Geometry: final body of the model. Coordinates: model frame, mm. Face numbers are marked on the shaded views. A direction names the side the tool comes from. Give positions to 0.01 mm unless a question says otherwise; leave off trailing zeros. Order: outer loops, then holes, each group sorted by start corner. A loop starts at its lowest first (then second) coordinate and runs counter-clockwise, first axis right, second up. Notation, with made-up numbers: (4.5, 16.25) - (52.5, 16.25) arc R13 cw to (52.5, 24.25) - close; hole circle Ø5 at (-1, 53.25). An arc over 180 degrees is marked (long way). Write item = value, one per line. Start each with the question number.
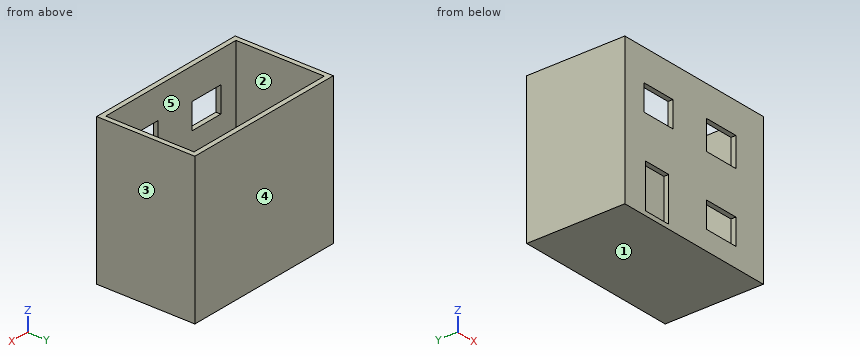
from build123d import *

# Parameters (mm, degrees)
F0_W     = 85.893087
F0_H     = 76.244824
F1_DEPTH = 50.8
F2_T     = -2.54
F3_W     = 17.883054
F3_H     = 13.338813
F3_W_2   = 18.097924
F3_H_2   = 15.061585
F3_H_3   = 13.338815
F3_W_3   = 14.340789
F3_H_4   = 22.664875
F4_DEPTH = 25.4


with BuildPart() as f1:
    # F0 (on Front) → F1 (new body)
    with BuildSketch(Plane.XZ):
        with Locations((2.00025, -38.122412)):
            Rectangle(F0_W, F0_H)
    extrude(amount=F1_DEPTH)

    # F2
    f2_openings = [f1.faces().sort_by_distance(p)[0] for p in [
        (2.00025, -25.4, 0),
    ]]
    offset(amount=F2_T, openings=f2_openings)

    # F3 (on face) → F4 (cut)
    with BuildSketch(Plane.XZ.offset(50.8)):
        with Locations((-20.056449, -22.847423)):
            Rectangle(F3_W, F3_H)
        with Locations((18.888849, -23.377542)):
            Rectangle(F3_W_2, F3_H_2)
        with Locations((18.888849, -59.610495)):
            Rectangle(F3_W_2, F3_H_3)
        with Locations((-20.887177, -62.660388)):
            Rectangle(F3_W_3, F3_H_4)
    extrude(amount=-F4_DEPTH, mode=Mode.SUBTRACT)


solid = f1.part
Q1. Contact query for a flat-ended pin moving along its axis: pin 1 (4.5 mm diameter, centred on x = -20.5, y = -34, fed in from +Z). Output: stop coordinate, or through.
Q2. Material intervals for line 1 along X through (y, z) = (-10, -23); line 2 along Y through (x, z) = (9, -44); line 3 along Z through (x, y) = (-17.5, -26.5), sorted ascending. Write a range as from..to.
Q3. Section A-A, the plane x = 13. Return the cut outline in (y, z).
Q4. Section B-B, the plane z = -62. Return the cut outline in (x, y), then the cut area to 3 significant figures.
Q5. Section C-C, the plane y = -23. Return the cut outline in (x, z).
Q6. Set-up query: the marked faces 1 and 2. Return all of +Z, -Z, +X, -X, +Y, -Y with unobstructed straight access to the full face (end or side cutting, diameter ignored); none if empty.
Q7. Pull-direction query (Y, two-part tool) for the marked faces 3, 4 and 5; classes: +Y half, -Y half, draft (parallel to the pull), parting line (faces both ways), or undercut.
Q8. Section D-D, the plane x = -5.5. Return the cut outline in (y, z).
The answers:
q1.pin_1 = -73.99
q2.line_1 = -40.95..-38.41, 42.41..44.95
q2.line_2 = -50.8..-48.26, -2.54..0
q2.line_3 = -76.24..-73.99
q3.outline = (-50.8, -76.24) - (0, -76.24) - (0, 0) - (-2.54, 0) - (-2.54, -73.7) - (-48.26, -73.7) - (-48.26, -66.28) - (-50.8, -66.28) - close; (-50.8, -52.94) - (-48.26, -52.94) - (-48.26, -30.91) - (-50.8, -30.91) - close; (-50.8, -15.85) - (-48.26, -15.85) - (-48.26, 0) - (-50.8, 0) - close
q4.outline = (-40.95, -50.8) - (-28.06, -50.8) - (-28.06, -48.26) - (-38.41, -48.26) - (-38.41, -2.54) - (42.41, -2.54) - (42.41, -48.26) - (27.94, -48.26) - (27.94, -50.8) - (44.95, -50.8) - (44.95, 0) - (-40.95, 0) - close; (-13.72, -50.8) - (9.84, -50.8) - (9.84, -48.26) - (-13.72, -48.26) - close
q4.area = 586 mm²
q5.outline = (-40.95, -76.24) - (44.95, -76.24) - (44.95, 0) - (42.41, 0) - (42.41, -73.7) - (-38.41, -73.7) - (-38.41, 0) - (-40.95, 0) - close
q6.face_1 = -Z, +X, -X, +Y, -Y
q6.face_2 = +Z
q7.face_3 = draft
q7.face_4 = +Y half
q7.face_5 = undercut
q8.outline = (-50.8, -76.24) - (0, -76.24) - (0, 0) - (-2.54, 0) - (-2.54, -73.7) - (-48.26, -73.7) - (-48.26, 0) - (-50.8, 0) - close
